Build history of the part. All positions in model axes, mm. Face numbers are marked on the shaded views. A direction names the side the tool comes from. Coordinates: 2 decimals unless noted, no trailing zeros. Order: outer loops, then holes, each group sorted by start corner. A loop starts at its lowest first (then second) coordinate and runs counter-clockwise, first axis right, second up. Notation, with made-up numbers: (-10.5, 15) - (37.5, 15) arc R28 cw to (37.5, 52) - close; hole circle Ø7 at (-9, 3.25). An arc over 180 degrees is marked (long way). One line per item, written item: value.
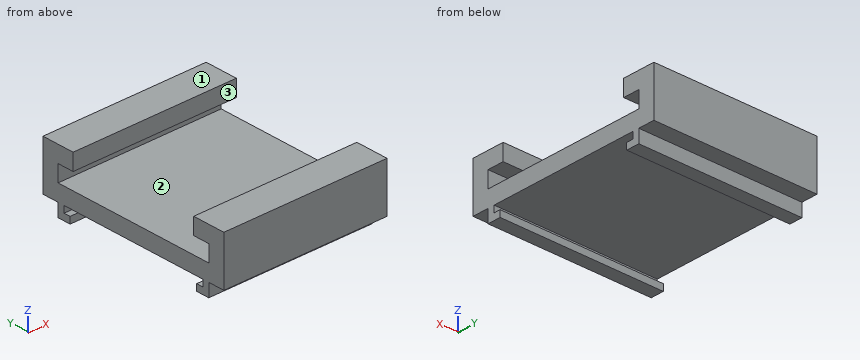
Autodesk Inventor part; units mm, degrees
ref_plane "YZ Plane" through (0, 0, 0) normal (1, 0, 0) x (0, 1, 0)
ref_plane "XZ Plane" through (0, 0, 0) normal (0, 1, 0) x (-1, 0, 0)
ref_plane "XY Plane" through (0, 0, 0) normal (0, 0, 1) x (1, 0, 0)
sketch "Sketch1" plane through (0, 0, 0) normal (0, 0, 1) x (1, 0, 0)
  line L0 (-25, 30) -> (25, 30)
  line L1 (25, 30) -> (25, -30)
  line L2 (25, -30) -> (-25, -30)
  line L3 (-25, -30) -> (-25, 30)
  point P0 (0, 0)
  dimension "d0" = 50
  dimension "d1" = 60
  dimension "d2" = 30
  dimension "d3" = 25
extrude "Extrusion1" add sketch "Sketch1" along normal blind 5
sketch "Sketch2" plane through (0, 0, 5) normal (0, 0, 1) x (1, 0, 0)
  line L0 (-25, 30) -> (-25, -30)
  line L1 (-25, 25) -> (25, 25)
  line L2 (25, -30) -> (25, 30)
  line L3 (25, 30) -> (-25, 30)
  point P0 (0, 0)
  dimension "d6" = 5
extrude "Extrusion2" add sketch "Sketch2" along normal blind 10
sketch "Sketch3" plane through (0, 0, 5) normal (0, 0, 1) x (1, 0, 0)
  line L0 (-25, -30) -> (-25, 30)
  line L1 (-25, -25) -> (25, -25)
  line L2 (25, 30) -> (25, -30)
  line L3 (-25, -30) -> (25, -30)
  point P0 (0, 0)
  dimension "d9" = 5
extrude "Extrusion3" add sketch "Sketch3" along normal blind 10
sketch "Sketch4" plane through (-25, -25, 5) normal (0, 1, 0) x (1, 0, 0)
  line L0 (0, 5) -> (0, -10)
  line L1 (0, -5) -> (50, -5)
  line L2 (50, 5) -> (50, -10)
  line L3 (0, -10) -> (50, -10)
  point P0 (25, 5)
  dimension "d12" = 5
extrude "Extrusion4" add sketch "Sketch4" along normal blind 5
sketch "Sketch5" plane through (-25, 25, 5) normal (0, -1, 0) x (1, 0, 0)
  line L0 (0, -5) -> (0, 10)
  line L1 (0, 5) -> (50, 5)
  line L2 (50, -5) -> (50, 10)
  line L3 (50, 10) -> (0, 10)
  point P0 (25, -5)
  dimension "d15" = 5
extrude "Extrusion5" add sketch "Sketch5" along normal blind 5
sketch "Sketch6" plane through (0, 0, 0) normal (0, 0, -1) x (-1, 0, 0)
  line L0 (-25, 30) -> (-25, -30)
  line L1 (25, -30) -> (25, 30)
  line L2 (-25, 25) -> (25, 25)
  line L3 (25, 25) -> (25, 23)
  line L4 (25, 23) -> (-25, 23)
  line L5 (-25, 23) -> (-25, 25)
  line L6 (25, 30) -> (-25, 30)
  point P0 (0, 0)
  dimension "d18" = 2
  dimension "d19" = 5
extrude "Extrusion6" add sketch "Sketch6" along normal blind 4 contours L2 L1 L4 L0
sketch "Sketch7" plane through (0, 0, 0) normal (0, 0, -1) x (-1, 0, 0)
  line L0 (-25, 23) -> (-25, -30)
  line L1 (25, -30) -> (25, 23)
  line L2 (-25, -25) -> (25, -25)
  line L3 (25, -25) -> (25, -23)
  line L4 (25, -23) -> (-25, -23)
  line L5 (-25, -23) -> (-25, -25)
  line L6 (-25, -30) -> (25, -30)
  point P0 (0, 0)
  dimension "d22" = 2
  dimension "d23" = 5
extrude "Extrusion7" add sketch "Sketch7" along normal blind 4 contours L4 L1 L2 L0
sketch "Sketch8" plane through (-25, 23, 0) normal (0, -1, 0) x (1, 0, 0)
  point P0 (25, 0)
sketch "Sketch9" plane through (-25, 23, 0) normal (0, -1, 0) x (1, 0, 0)
  line L0 (50, 0) -> (50, -4)
  line L1 (0, 0) -> (0, -4)
  line L2 (50, -4) -> (0, -4)
  line L3 (0, -4) -> (0, -2)
  line L4 (0, -2) -> (50, -2)
  line L5 (50, -2) -> (50, -4)
  point P0 (25, 0)
extrude "Extrusion8" add sketch "Sketch9" along normal blind 2
sketch "Sketch10" plane through (-25, -23, 0) normal (0, 1, 0) x (1, 0, 0)
  line L0 (0, 0) -> (0, 4)
  line L1 (50, 0) -> (50, 4)
  line L2 (0, 4) -> (50, 4)
  line L3 (50, 4) -> (50, 2)
  line L4 (50, 2) -> (0, 2)
  line L5 (0, 2) -> (0, 4)
  point P0 (25, 0)
extrude "Extrusion9" add sketch "Sketch10" along normal blind 2
properties part number "Substrategrip0degreesThick"
1. Band-saw the part on C-C, the plane y = -26. Give the cut face in (x, z).
Values found:
outline: (-25, 0) - (25, 0) - (25, 15) - (-25, 15) - close
2. 3-axis set-ups, long thin cutter, end or side, ignore diameter. For the marked faces 1, 2 and 3: which of +Z, -Z, +X, -X, +Y, -Y reach the whole face in a straight line?
Values found:
face 1: +Z, +X, -X, +Y, -Y
face 2: +X, -X
face 3: +Z, +X, -X
3. Band-saw the part on D-D, the plane y = 16. Give the cut face in (x, z), and give its area (3 significant figures).
Values found:
outline: (-25, 0) - (25, 0) - (25, 5) - (-25, 5) - close
area: 250 mm2
4. Flat gauge pins, fed straight in: P1, Ø2, axis at x = -9, z = -3, coming from the +Y side; P2, Ø1.2, axis at x = 5.5, z = -1.5, coming from the -Y side; P3, Ø23, axis at x = 0.5, y = 1, coming from the -Z side. Where does each tip first touch, or does it go through?
Values found:
P1: stops at y = 25
P2: stops at y = -25
P3: stops at z = 0
5. Band-saw the part on A-A, the plane z = 12.75. Give the cut face in (x, y).
Values found:
outline: (-25, -30) - (25, -30) - (25, -20) - (-25, -20) - close; (-25, 20) - (25, 20) - (25, 30) - (-25, 30) - close
6. Band-saw the part on B-B, the plane x = -18. Give the cut face in (y, z), and give its area (3 significant figures).
Values found:
outline: (-30, 0) - (-25, 0) - (-25, -4) - (-21, -4) - (-21, -2) - (-23, -2) - (-23, 0) - (23, 0) - (23, -2) - (21, -2) - (21, -4) - (25, -4) - (25, 0) - (30, 0) - (30, 15) - (20, 15) - (20, 10) - (25, 10) - (25, 5) - (-25, 5) - (-25, 10) - (-20, 10) - (-20, 15) - (-30, 15) - close
area: 474 mm2
7. Probe line 1 along Z through (x, y) = (22, 22.5); line 2 along Y through (x, z) = (17, 5.5); line 3 along Y through (x, z) = (11, 10.75). List the from-to ranges inside material, lowest first.
Values found:
line 1: z = -4 to -2, 0 to 5, 10 to 15
line 2: y = -30 to -25, 25 to 30
line 3: y = -30 to -20, 20 to 30
